Build history of the part. All positions in model axes, mm. A direction names the side the tool comes from. Coordinates: 2 decimals unless noted, no trailing zeros. Write each loop counter-clockwise with the first axis right and the second up, starting at its lowest first coordinate (ties: lowest second). Pieces come first, ordered by that corner, then holes.
```python
from build123d import *

# Parameters (mm, degrees)
F0_W     = 5
F0_H     = 80
F1_DEPTH = 50
F2_DEPTH = 39
F4_D     = 10


with BuildPart() as f1:
    # F0 (on Top) → F1 (new body)
    with BuildSketch(Plane.XY):
        Polygon((-42.571511, -141.256928), (0, -141.256928), (42.571511, -141.256928), (75.937726, -53.33484), (104.205489, 154.886812), (98.816866, 228.730714), (72.5, 228.730714), (72.5, 148.730714), (67.5, 148.730714), (27, -69.269286), (0, -69.269286), (-27, -69.269286), (-67.5, 148.730714), (-72.5, 148.730714), (-72.5, 228.730714), (-98.816866, 228.730714), (-104.205489, 154.886812), (-75.937726, -53.33484), align=None)
        with Locations((70, 188.730714)):
            Rectangle(F0_W, F0_H)
        with Locations((-70, 188.730714)):
            Rectangle(F0_W, F0_H)
    extrude(amount=F1_DEPTH)

    # F0 (on Top) → F2 (join)
    with BuildSketch(Plane.XY):
        with Locations((-70, 188.730714)):
            Rectangle(F0_W, F0_H)
        with Locations((70, 188.730714)):
            Rectangle(F0_W, F0_H)
    extrude(amount=-F2_DEPTH)

    # F4 (through all)
    with Locations(Plane.YZ.offset(72.5)):
        with Locations((198.730714, -29)):
            Hole(F4_D / 2)


solid = f1.part
```
1. Saw through at B-B on z = -8. List the corners of the cut face in (x, y).
Computed values:
outline: (-72.5, 148.73) - (-67.5, 148.73) - (-67.5, 228.73) - (-72.5, 228.73) - close; (67.5, 148.73) - (72.5, 148.73) - (72.5, 228.73) - (67.5, 228.73) - close
2. Saw through at C-C on y = 170.5. List the corners of the cut face in (x, z), plus the area to 3 significant figures.
Computed values:
outline: (-103.07, 0) - (-72.5, 0) - (-72.5, -39) - (-67.5, -39) - (-67.5, 50) - (-103.07, 50) - close; (67.5, -39) - (72.5, -39) - (72.5, 0) - (103.07, 0) - (103.07, 50) - (67.5, 50) - close
area: 3,950 mm2
3. 3-axis set-ups, long thin cutter, end or side, ignore diameter. For faces 1 (the face through (67.5, 188, 5)), 2 (the face through (59.02, -97.91, 24.65)): which of +Z, -Z, +X, -X, +Y, -Y reach the whole face in a straight line?
Computed values:
face 1: +Z, -Z, +Y
face 2: +Z, -Z, +X, -Y
4. Probe line 1 along Z through (x, y) = (-90, 112); line 2 along X through (y, z) = (-11, 41.5); line 3 along X through (y, z) = (25, 18.5). List the from-to ranges inside material, lowest first.
Computed values:
line 1: z = 0 to 50
line 2: x = -81.69 to -37.83, 37.83 to 81.69
line 3: x = -86.57 to -44.51, 44.51 to 86.57
5. Saw through at D-D on z = 25. List the corners of the cut face in (x, y).
Computed values:
outline: (-104.21, 154.89) - (-75.94, -53.33) - (-42.57, -141.26) - (42.57, -141.26) - (75.94, -53.33) - (104.21, 154.89) - (98.82, 228.73) - (67.5, 228.73) - (67.5, 148.73) - (27, -69.27) - (-27, -69.27) - (-67.5, 148.73) - (-67.5, 228.73) - (-98.82, 228.73) - close
6. Flat gauge pins, fed straight in: pin 1 (2.5 mm diameter, centred on x = 71, z = -11.5, fed in from -Y); pin 2 (12 mm diameter, centred on y = 153.5, z = -25, fed in from +X); pin 3 (10 mm diameter, centred on y = 173.5, z = -2, fed in from -X). Where does each tip first touch, or does it go through?
Computed values:
pin 1: stops at y = 148.73
pin 2: stops at x = 72.5
pin 3: stops at x = -103.18
7. Mould opens along X. For faces 3 (the face through (47.534, 41.257, 24.65)), 4 (the face through (-72.5, 188, -19)), 5 (the face through (72.5, 188, -19)) say: +X half, -X half, draft (parallel to the pull), parting line (faces both ways), or undercut.
Computed values:
face 3: undercut
face 4: -X half
face 5: +X half
8. Saw through at A-A on z = -29. List the corners of the cut face in (x, y), plus the area to 3 significant figures.
Computed values:
outline: (-72.5, 148.73) - (-67.5, 148.73) - (-67.5, 193.73) - (-72.5, 193.73) - close; (-72.5, 203.73) - (-67.5, 203.73) - (-67.5, 228.73) - (-72.5, 228.73) - close; (67.5, 148.73) - (72.5, 148.73) - (72.5, 193.73) - (67.5, 193.73) - close; (67.5, 203.73) - (72.5, 203.73) - (72.5, 228.73) - (67.5, 228.73) - close
area: 700 mm2
